Drawing for the job (mm, zero at the part's lowest x, y, z). A direction names the side the tool comes from. Coordinates: 2 decimals unless noted, no trailing zeros. Loops run counter-clockwise (first coordinate to the right, second up) from the corner with the lowest first, then second, coordinate; pieces in that order, holes last. Notation, with made-up numbers: (-29, -40) - (-13, -40) arc R26 ccw to (-13, -3) - close; hole circle Ø3 at (-2.75, 65). An arc over 180 degrees is marked (long way). One line per item, written item: value.
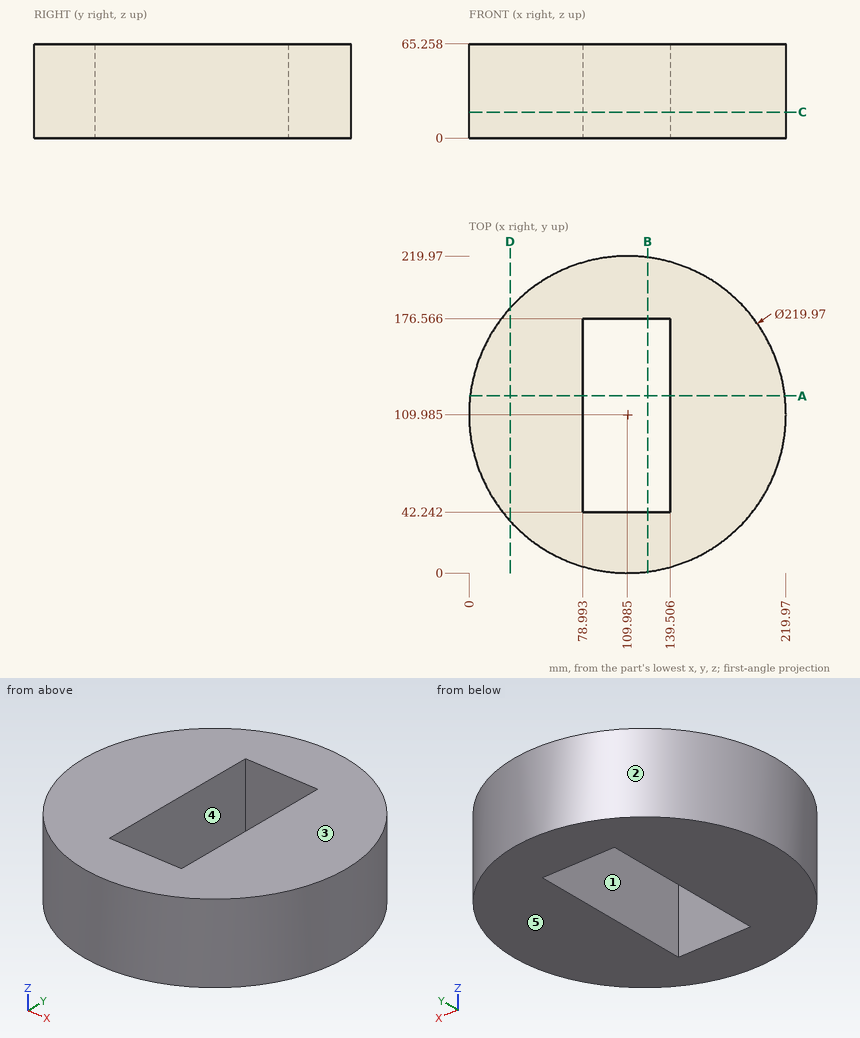
Item 1: Tool access for the marked faces 4 and 5: list every direction of +Z, -Z, +X, -X, +Y, -Y with a clear straight run to the whole face (end or side of a thin tool).
Check result:
face 4: +Z, -Z
face 5: -Z, +X, -X, +Y, -Y
Item 2: Probe probe 1 along X at (y, z) = (111.5, 29.5); probe 2 along Y at (x, z) = (107, 32); probe 3 along Y at (x, z) = (110, 16). List the from-to ranges inside material, lowest first. Write a range as from..to.
Check result:
probe 1: x = 0.01..78.99, 139.51..219.96
probe 2: y = 0.04..42.24, 176.57..219.93
probe 3: y = 0..42.24, 176.57..219.97
Item 3: Cut at D-D, the plane x = 28.5. Write the cut outline in (y, z) (1 decimal).
Check result:
outline: (36.1, 0) - (183.9, 0) - (183.9, 65.3) - (36.1, 65.3) - close
Item 4: Drop flat-ended pins along their axis: P1, Ø1, axis at y = 138.5, z = 32.5, coming from the +X side; P2, Ø1, axis at x = 103.5, z = 41.5, coming from the +Y side; P3, Ø8, axis at y = 192.5, z = 49, coming from the +X side (1 decimal); P4, Ø6, axis at x = 150, y = 93.5, coming from the -Z side. Give the stop position or say it passes through.
Check result:
P1: stops at x = 216.34
P2: stops at y = 219.81
P3: stops at x = 187
P4: stops at z = 0
Item 5: Cut at A-A, the plane y = 123. Write the cut outline in (x, z), then the cut area to 3 significant figures.
Check result:
outline: (0.77, 0) - (78.99, 0) - (78.99, 65.26) - (0.77, 65.26) - close; (139.51, 0) - (219.2, 0) - (219.2, 65.26) - (139.51, 65.26) - close
area: 10,300 mm^2
Item 6: Pull direction Y, two halves, no side cores. Call the marked faces 1, 2 and 3: released by +Y, released by -Y, zero draft, split by the parting line, or undercut.
Check result:
face 1: undercut
face 2: split by the parting line
face 3: zero draft
Item 7: Cut at C-C, the plane z = 18. Write the cut outline in (x, y) (1 decimal).
Check result:
outline: circle Ø220 at (110, 110); hole (79, 42.2) - (139.5, 42.2) - (139.5, 176.6) - (79, 176.6) - close
Item 8: Cut at B-B, the plane x = 124. Write the cut outline in (y, z).
Check result:
outline: (0.9, 0) - (42.24, 0) - (42.24, 65.26) - (0.9, 65.26) - close; (176.57, 0) - (219.07, 0) - (219.07, 65.26) - (176.57, 65.26) - close
